CAD build for the part. Positions are in the model's coordinates, mm. A direction names the side the tool comes from. Coordinates: 2 decimals unless noted, no trailing zeros. Loops run counter-clockwise (first coordinate to the right, second up) from the corner with the lowest first, then second, coordinate; pieces in that order, holes last. Notation, with made-up numbers: (67, -13) -> (112, -13) arc R17 ccw to (112, -5) -> close; hole circle Ø7 at (20, 57.25). An arc over 180 degrees is marked (long way). Answer as CSV lines item,"result". Start each with the question number.
```python
from build123d import *

# Parameters (mm, degrees)
F1_DEPTH = 10
F2_W     = 5.5
F2_H     = 5.5
F3_DEPTH = 5.5
F4_W     = 5.5
F4_H     = 5.5
F5_DEPTH = 5.5
F6_R     = 1


with BuildPart() as f1:
    # F0 (on Front) → F1 (new body)
    with BuildSketch(Plane.XZ):
        Polygon((11, 0), (0, 0), (-31.233847, -62.645405), (-31.233847, -69.645405), (-6.233847, -69.645405), (-9.894388, -27.805228), (11, -32), align=None)
    extrude(amount=F1_DEPTH)

    # F2 (on face) → F3 (cut)
    with BuildSketch(Plane(origin=(-31.233847, 0, 0), x_dir=(0, -1, 0), z_dir=(-1, 0, 0))):
        with Locations((5, -66.145405)):
            Rectangle(F2_W, F2_H)
    extrude(amount=-F3_DEPTH, mode=Mode.SUBTRACT)

    # F4 (on face) → F5 (cut)
    with BuildSketch(Plane.XY):
        with Locations((5.5, -5)):
            Rectangle(F4_W, F4_H)
    extrude(amount=-F5_DEPTH, mode=Mode.SUBTRACT)

    # F6
    f6_edges = [f1.edges().sort_by_distance(p)[0] for p in [
        (0.552806, -10, -29.902614),
        (-18.733847, -10, -69.645405),
        (-8.064118, -10, -48.725317),
        (11, -10, -16),
    ]]
    fillet(f6_edges, radius=F6_R)


solid = f1.part
```
Q1. Saw through at D-D (y = -7). List the corners of the cut face in (x, z).
Q2. Probe probe 1 along X at (y, z) = (-6, -3); probe 2 along Z at (x, y) = (7.5, -2.5); probe 3 along X at (y, z) = (-5.5, -5). List the from-to ranges inside material, lowest first. Write a range as from..to.
Q3. Saw through at B-B (z = -4). List the corners of the cut face in (x, y).
Q4. Which spindle directions (+Z, -Z, +X, -X, +Y, -Y) get a long thin tool onto all of the face, cutting with end or side? Do faces 5 (the flat face through (-29, -5, -63.395)), 6 (the flat face through (8.25, -5, -3)), 7 (the cylindrical face through (0.11, -9.71, -29.51)), 8 (the flat face through (-11, -10, -34)). Say none if no direction does.
Q5. Saw through at C-C (x = -27). List the corners of the cut face in (y, z), and give its area (3 significant figures).
Q6. Saw through at A-A (y = -1.5). List the corners of the cut face in (x, z).
Q7. Pin check, flat tips, straight feed: pin 1 Ø3 at (x, y) = (-29.5, -6.5) entering from +Z; pin 2 Ø1.6 at (x, z) = (5, -2.5) entering from +Y; pin 3 Ø1.5 at (y, z) = (-6.5, -47.5) entering from -X; pin 4 Ø3 at (x, y) = (4.5, -5.5) entering from +Z. Stop position of each tip, or through.
Q8. Two-plate mould, pull along Z, no slides. Class faces 1 (the flat face through (-15.398, -4.93, -30.884)), 2 (the flat face through (-29, -5, -68.895)), 3 (the flat face through (-25.734, -5, -66)), 4 (the flat face through (-31.234, -5, -63)): pulls with the +Z half, pulls with the -Z half, needs draft (parallel to the pull), parting line crosses it, or undercut.
Ans:
1,outline,"(-31.23, -69.65) -> (-6.23, -69.65) -> (-9.89, -27.81) -> (11, -32) -> (11, 0) -> (8.25, 0) -> (8.25, -5.5) -> (2.75, -5.5) -> (2.75, 0) -> (0, 0) -> (-31.23, -62.65) -> (-31.23, -63.4) -> (-25.73, -63.4) -> (-25.73, -68.9) -> (-31.23, -68.9) -> close"
2,probe 1,"x = -1.5..2.75, 8.25..11"
2,probe 2,"z = -31.3..-5.5"
2,probe 3,"x = -2.49..2.75, 8.25..11"
3,outline,"(-1.99, -10) -> (10, -10) arc R1 ccw to (11, -9) -> (11, 0) -> (-1.99, 0) -> close; hole (2.75, -7.75) -> (8.25, -7.75) -> (8.25, -2.25) -> (2.75, -2.25) -> close"
4,face 5,"-X"
4,face 6,"+Z"
4,face 7,"-Y"
4,face 8,"+Z, -Z, +X, -X, -Y"
5,outline,"(-10, -68.65) arc R1 ccw to (-9, -69.65) -> (0, -69.65) -> (0, -54.15) -> (-10, -54.15) -> close; hole (-7.75, -68.9) -> (-2.25, -68.9) -> (-2.25, -63.4) -> (-7.75, -63.4) -> close"
5,area,"124 mm²"
6,outline,"(-31.23, -69.65) -> (-6.23, -69.65) -> (-9.89, -27.81) -> (11, -32) -> (11, 0) -> (0, 0) -> (-31.23, -62.65) -> close"
7,pin 1,"stops at z = -56.16"
7,pin 2,"stops at y = 0"
7,pin 3,"stops at x = -24.06"
7,pin 4,"stops at z = -5.5"
8,face 1,"pulls with the +Z half"
8,face 2,"undercut"
8,face 3,"undercut"
8,face 4,"needs draft"
